Source: CAD feature listing. Evaluate the final solid. Frame: model axes, mm. Face numbers are marked on the shaded views. A direction names the side the tool comes from. Coordinates: 2 decimals unless noted, no trailing zeros. Loops run counter-clockwise (first coordinate to the right, second up) from the corner with the lowest first, then second, coordinate; pieces in that order, holes last. Notation, with made-up numbers: M 19.5,-2 L 56.5,-2 A25 cw 56.5,20 Z; hole C 80,75.25 d4. An arc over 180 degrees is marked long. Write each question's results on one line, items separated by ' | '. Start each with the question number.
from build123d import *

# Parameters (mm, degrees)
SKETCH_1_W                = 63
SKETCH_1_H                = 13
EXTRUDE_1_DEPTH           = 10
HOLE_WIZARD_1_D           = 6.6
HOLE_WIZARD_1_CBORE_D     = 11
HOLE_WIZARD_1_CBORE_DEPTH = 6.8
MM_1_D                    = 4
MM_1_DEPTH                = 5
MM_1_TIP                  = 1.201721238
CUT_EXTRUDE_1_DEPTH       = 5
HOLE_WIZARD_M2_1_D        = 1.6
SKETCH_9_W                = 11.9
SKETCH_9_H                = 9.8
CUT_EXTRUDE_2_DEPTH       = 36.514081714


with BuildPart() as part:
    # 草图1 → 凸台-拉伸1 (new body)
    with BuildSketch(Plane(origin=(0, 0, 0), x_dir=(1, 0, 0), z_dir=(0, 1, 0))):
        Rectangle(SKETCH_1_W, SKETCH_1_H)
    extrude(amount=EXTRUDE_1_DEPTH)

    # 打孔尺寸(%根据)内六角圆柱头螺钉的类型1 (through all)
    with Locations(Plane(origin=(-25, 10, 0), x_dir=(0, 0, 1), z_dir=(0, 1, 0))):
        with Locations((0, 0), (0, 50)):
            CounterBoreHole(HOLE_WIZARD_1_D / 2, HOLE_WIZARD_1_CBORE_D / 2, HOLE_WIZARD_1_CBORE_DEPTH)

    # 大小mm 暗销孔1
    with Locations(Plane(origin=(-15, 0, 0), x_dir=(0, 0, -1), z_dir=(0, -1, 0))):
        with Locations((0, 0)):
            Hole(MM_1_D / 2, depth=MM_1_DEPTH)
            with Locations((0, 0, -(MM_1_DEPTH + MM_1_TIP / 2))):  # 118° drill point
                Cone(0, MM_1_D / 2, MM_1_TIP, mode=Mode.SUBTRACT)

    # 草图6 → 切除-拉伸1 (cut)
    with BuildSketch(Plane.XZ):
        with BuildLine():
            Line((14.5, 2), (15.5, 2))
            ThreePointArc((15.5, 2), (17.5, 0), (15.5, -2))
            Line((15.5, -2), (14.5, -2))
            ThreePointArc((14.5, -2), (12.5, 0), (14.5, 2))
        make_face()
    extrude(amount=-CUT_EXTRUDE_1_DEPTH, mode=Mode.SUBTRACT)

    # M2 螺纹孔1 (through all)
    with Locations(Plane.ZX.offset(10)):
        with Locations((0, 0)):
            Hole(HOLE_WIZARD_M2_1_D / 2)

    # 草图9 → 切除-拉伸2 (cut, through all)
    with BuildSketch(Plane.XY.offset(6.5)):
        with Locations((0, 4.9)):
            Rectangle(SKETCH_9_W, SKETCH_9_H)
    extrude(amount=-CUT_EXTRUDE_2_DEPTH, mode=Mode.SUBTRACT)


solid = part.part
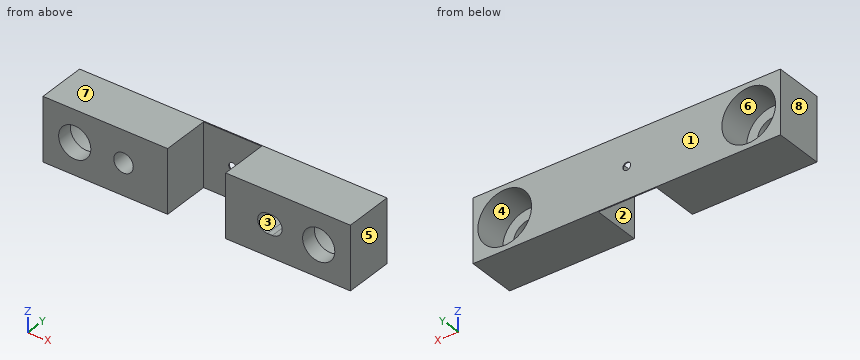
Item 1: Line query: probe 1 along X at (y, z) = (7.5, 0); probe 2 along X at (y, z) = (0.5, 5.5); probe 3 along X at (y, z) = (3.75, -4). Output: solid intervals per line, ascending.
Item 2: Access query for the marked faces 1, 2, 3 and 4. Directions: +Z, -Z, +X, -X, +Y, -Y. A direction counts if a zero-diameter tool reaches every point of the face in a straight line with its end or side. Return the directions, or none.
Item 3: Cut plane D-D (y = 4). Output: boundary loops of the cut face in (x, z), then the cut area to 3 significant figures.
Item 4: Cut plane C-C (z = 2.75). Output: boundary loops of the cut face in (x, y), then the cut area to 3 significant figures.
Item 5: Cut plane B-B (x = -25). Output: boundary loops of the cut face in (y, z), then the cut area to 3 significant figures.
Item 6: Mould query, pull axis X, two halves, no side actions, for the marked faces 5, 6, 7 and 8. Classes: +X half, -X half, draft (parallel to the pull), parting line (faces both ways), or undercut.
Item 7: Cut plane A-A (y = 0.75). Output: boundary loops of the cut face in (x, z).
Item 8: First-contact query: pin 1 Ø2 at (x, z) = (14.5, -0.5) entering from -Y; pin 2 Ø6 at (x, z) = (25, 0) entering from +Y. Flat tips, straight axial feed; report the tip coordinate or a pass-through.
Response values:
1) probe 1: x = -31.5 to -30.5, -19.5 to -5.95, 5.95 to 19.5, 30.5 to 31.5 | probe 2: x = -31.5 to -5.95, 5.95 to 31.5 | probe 3: x = -31.5 to -28.77, -21.23 to -5.95, 5.95 to 21.23, 28.77 to 31.5
2) face 1: +Z, -Z, +X, -X, +Y | face 2: +Z, -Z, -Y | face 3: -Y | face 4: +Y
3) outline: M -31.5,-6.5 L -5.95,-6.5 L -5.95,6.5 L -31.5,6.5 Z; M 5.95,-6.5 L 31.5,-6.5 L 31.5,6.5 L 5.95,6.5 Z; hole C -25,0 d11; hole C -15,0 d4; hole M 14.5,-2 L 15.5,-2 A2 ccw 15.5,2 L 14.5,2 A2 ccw Z; hole C 25,0 d11 | area: 445 mm2
4) outline: M -31.5,0 L -26.82,0 L -26.82,3.2 L -29.76,3.2 L -29.76,10 L -31.5,10 Z; M -23.18,0 L -5.95,0 L -5.95,9.8 L 5.95,9.8 L 5.95,0 L 23.18,0 L 23.18,3.2 L 20.24,3.2 L 20.24,10 L -20.24,10 L -20.24,3.2 L -23.18,3.2 Z; M 26.82,0 L 31.5,0 L 31.5,10 L 29.76,10 L 29.76,3.2 L 26.82,3.2 Z | area: 360 mm2
5) outline: M 0,-6.5 L 10,-6.5 L 10,-5.5 L 3.2,-5.5 L 3.2,-3.3 L 0,-3.3 Z; M 0,3.3 L 3.2,3.3 L 3.2,5.5 L 10,5.5 L 10,6.5 L 0,6.5 Z | area: 34.1 mm2
6) face 5: +X half | face 6: undercut | face 7: draft | face 8: -X half
7) outline: M -31.5,-6.5 L -5.95,-6.5 L -5.95,6.5 L -31.5,6.5 Z; M 5.95,-6.5 L 31.5,-6.5 L 31.5,6.5 L 5.95,6.5 Z; hole C -25,0 d6.6; hole C -15,0 d4; hole M 14.5,-2 L 15.5,-2 A2 ccw 15.5,2 L 14.5,2 A2 ccw Z; hole C 25,0 d6.6
8) pin 1: stops at y = 5 | pin 2: passes through
